from build123d import *

# Parameters (mm, degrees)
SKETCH2_R          = 6.35
SKETCH2_R_2        = 3.175
CIRCULAR_CUT_DEPTH = 110.433918417
CIRPATTERN_COUNT   = 12
SLOT_CUT_DEPTH     = 110.433918417


with BuildPart() as part:
    # Sketch1 → Revolve 2 (revolve)
    with BuildSketch(Plane.XY, mode=Mode.PRIVATE) as revolve_2_sk:
        Polygon((0, 0), (0, 76.2), (-25.4, 76.2), (-25.4, 69.85), (-6.35, 69.85), (-6.35, 43.954479769), (-19.05, 43.954479769), (-19.05, 38.1), (-6.35, 38.1), (-6.35, 0), align=None)
    revolve(revolve_2_sk.sketch.rotate(Axis((-6.35, 0, 0), (1, 0, 0)), 90), axis=Axis((-6.35, 0, 0), (1, 0, 0)))

    # Sketch2 → Circular Cut (cut, through all)
    with BuildSketch(Plane.ZY.offset(6.35)):
        with Locations((57.15, 0)):
            Circle(SKETCH2_R)
        with Locations((25.4, 0)):
            Circle(SKETCH2_R_2)
    circular_cut = extrude(amount=-CIRCULAR_CUT_DEPTH, mode=Mode.SUBTRACT)

    # CirPattern: Circular Cut ×12 about axis
    cirpattern_axis = Axis((0, 0, 0), (1, 0, 0))
    for i in range(1, CIRPATTERN_COUNT):
        add(circular_cut.rotate(cirpattern_axis, i * 360 / CIRPATTERN_COUNT), mode=Mode.SUBTRACT)

    # Sketch5 → Slot Cut (cut, through all)
    with BuildSketch(Plane.ZY.offset(6.35)):
        with BuildLine():
            Line((-7.9375, 4.7625), (7.9375, 4.7625))
            ThreePointArc((7.9375, 4.7625), (12.7, 0), (7.9375, -4.7625))
            Line((7.9375, -4.7625), (-7.9375, -4.7625))
            ThreePointArc((-7.9375, -4.7625), (-12.7, 0), (-7.9375, 4.7625))
        make_face()
    extrude(amount=-SLOT_CUT_DEPTH, mode=Mode.SUBTRACT)


solid = part.part
The model under review builds one solid part; all positions refer to its coordinate system, in mm. A direction names the side the tool comes from. Coordinates: 2 decimals unless noted, no trailing zeros. Write each loop counter-clockwise with the first axis right and the second up, starting at its lowest first coordinate (ties: lowest second). Pieces come first, ordered by that corner, then holes. Notation, with made-up numbers: (2, 24.5) -> (8, 24.5) arc R26 cw to (8, 45.5) -> close; hole circle Ø6 at (-7.75, 64). An arc over 180 degrees is marked (long way). Answer in a Markdown table with one row per item.
1. We need section A-A, the plane x = -17.25. State the section outline as (y, z) points.
Answers below:
| item | result |
|---|---|
| outline | circle Ø152.4 at (0, 0); circle Ø87.91 at (0, 0); hole circle Ø139.7 at (0, 0); hole circle Ø76.2 at (0, 0) |
2. Draft analysis for pull direction Z (two halves, no side actions). For faces 1 (the flat face through (-25.4, 62, 34)), 2 (the cylindrical face through (-3.219, 0.279, 50.806)), state which applies: +Z half, -Z half, draft (parallel to the pull), parting line (faces both ways), or undercut.
Answers below:
| item | result |
|---|---|
| face 1 | draft |
| face 2 | undercut |
3. Clearance check with flat-ended pins moving along their axes: pin 1 Ø6 at (x, y) = (-9.5, 38.5) entering from -Z; pin 2 Ø2 at (x, z) = (-10, -29) entering from -Y; pin 3 Ø1 at (x, z) = (-5.5, -31) entering from +Y. State where each tip first meets the part, or that it passes through.
Answers below:
| item | result |
|---|---|
| pin 1 | stops at z = -67.43 |
| pin 2 | stops at y = -70.87 |
| pin 3 | stops at y = 69.83 |
4. We need section B-B, the plane z = -47.5. State the section outline as (x, y) points, and give its area (3 significant figures).
Answers below:
| item | result |
|---|---|
| outline | (-25.4, -59.58) -> (0, -59.58) -> (0, -34.6) -> (-6.35, -34.6) -> (-6.35, -51.21) -> (-25.4, -51.21) -> close; (-25.4, 51.21) -> (-6.35, 51.21) -> (-6.35, 34.6) -> (0, 34.6) -> (0, 59.58) -> (-25.4, 59.58) -> close; (-6.35, -22.55) -> (0, -22.55) -> (0, 22.55) -> (-6.35, 22.55) -> close |
| area | 922 mm^2 |
5. For faces 3 (the cylindrical face through (-3.2, 0.1, 12.7)), 4 (the cylindrical face through (-12.79, 42.91, -9.53)), list the 3-axis set-ups (+Z, -Z, +X, -X, +Y, -Y) from which the entire face can be reached by the end or side of a thin tool; tool diameter is ignored.
Answers below:
| item | result |
|---|---|
| face 3 | +X, -X |
| face 4 | -X |
6. We need section C-C, the plane y = 0. Give the number of separate pieces and of enclosed holes in the cut face, and give its area (3 significant figures).
Answers below:
| item | result |
|---|---|
| separate pieces | 6 |
| enclosed holes | 0 |
| area | 955 mm^2 |
7. Wall thickness on probe 1 along Y at (x, z) = (-6, -32.5); probe 2 along Z at (x, y) = (-13.5, 8.5); probe 3 along Z at (x, y) = (-3, -12.7): over which ranges is each line inside the solid? List them lowest first. Write a range as [from, to].
Answers below:
| item | result |
|---|---|
| probe 1 | y = [-68.92, -54.49], [-44.5, 44.5], [54.49, 68.92] |
| probe 2 | z = [-75.72, -69.33], [-43.12, -37.14], [37.14, 43.12], [69.33, 75.72] |
| probe 3 | z = [-75.13, -25.17], [-18.82, 18.82], [25.17, 75.13] |
